Input: dimensioned drawing with shaded views. Units: mm. Origin: part minimum x, y, z. Coordinates: 2 decimals unless noted, no trailing zeros. Write each loop counter-clockwise with the first axis right and the second up, starting at its lowest first coordinate (ties: lowest second). Pieces come first, ordered by that corner, then holes. Notation, with made-up numbers: M 61.25,8 L 100.25,8 A36 ccw 100.25,42 Z; hole C 44.25,67 d7. An arc over 180 degrees is marked long. Write each question's results on one line, items separated by ' | '. Start each with the question number.
1. Section query B-B, the plane x = 6.5. Output: boundary loops of the cut face in (y, z).
2. Section query C-C, the plane z = 2. Output: boundary loops of the cut face in (x, y).
3. Section query D-D, the plane x = 22. Output: boundary loops of the cut face in (y, z), and give its area (3 significant figures).
4. First-contact query: pin 1 (3 mm diameter, centred on y = 23, z = 3.5, fed in from -X); pin 2 (3 mm diameter, centred on y = 6, z = 5, fed in from +X). Flat tips, straight axial feed; report the tip coordinate or a pass-through.
5. Section query A-A, the plane y = 40.5. Output: boundary loops of the cut face in (x, z).
6. Pull-direction query (X, two-part tool) for the marked faces 1, 2 and 3; classes: +X half, -X half, draft (parallel to the pull), parting line (faces both ways), or undercut.
7. Ray query, probe 1 along Y at (x, z) = (16, 1.5); probe 2 along X at (y, z) = (37, 2); probe 3 along Y at (x, z) = (9, 2.75). Return the intervals inside material, ascending.
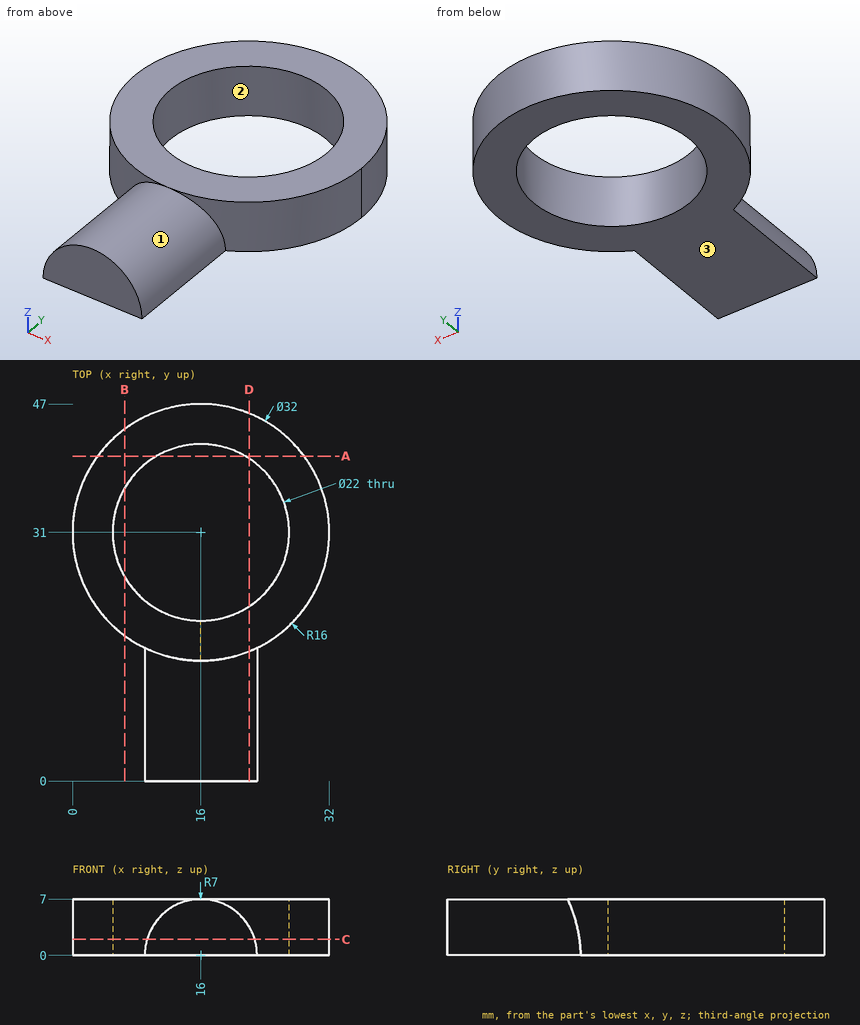
Answer:
1) outline: M 18.13,0 L 25.45,0 L 25.45,7 L 18.13,7 Z; M 36.55,0 L 43.87,0 L 43.87,7 L 36.55,7 Z
2) outline: M 9.29,0 L 22.71,0 L 22.71,16.47 A16 ccw long 9.29,16.47 Z; hole C 16,31 d22
3) outline: M 0,0 L 21.78,0 L 21.78,7 L 16.17,7 L 16.17,3.61 L 0,3.61 Z; M 40.22,0 L 45.83,0 L 45.83,7 L 40.22,7 Z | area: 137 mm^2
4) pin 1: x = 1.38 | pin 2: x = 22.06
5) outline: M 3.13,0 L 10.45,0 L 10.45,7 L 3.13,7 Z; M 21.55,0 L 28.87,0 L 28.87,7 L 21.55,7 Z
6) face 1: parting line | face 2: undercut | face 3: draft
7) probe 1: 0 to 20, 42 to 47 | probe 2: 1.17 to 6.78, 25.22 to 30.83 | probe 3: 16.61 to 22.51, 39.49 to 45.39
